Geometry: final body of the model. Coordinates: model frame, mm. A direction names the side the tool comes from. Give positions to 0.01 mm unless a question says otherwise; leave off trailing zeros. Write each loop counter-clockwise with the first axis right and the second up, starting at its lowest first coordinate (ties: lowest second). Pieces come first, ordered by that corner, then holes. Notation, with made-up numbers: M -35,-37 L -27,-37 A14 cw -27,-29 Z; hole C 31.25,26 d8. An arc over 180 degrees is marked long. Use a Markdown table: item, result. Add a question column.
(1) Material intervals for L1, parallel to Y at x = 0, z = 1.35; L2, parallel to Z at x = -14.5, y = 4.5; L3, parallel to X at y = 4, z = 0.3, sorted ascending.
(2) Cut plane B-B (y = -3.75). Output: boundary loops of the cut face in (x, z).
(3) Draft query along Y for faces 4 (the cylindrical face through (13.46, -1.36, 1.32)), 5 (the flat face through (0, -9, 1)), 6 (the flat face through (-11, 9, 1)). Return one class per face: released by +Y, released by -Y, zero draft, split by the parting line, or undercut.
(4) Pin query (flat end, axial travel): pin 1 Ø2.5 at (y, z) = (12.5, 2.5) entering from -X; pin 2 Ø1 at (y, z) = (7.5, 1.5) entering from +X; pin 3 Ø16 at (x, y) = (-6, -1) entering from +Z. Return the tip coordinate at first contact, or that it passes through.
(5) Reachability of faces 1 (the flat face through (8, 12, 2)), 2 (the flat face through (-12, 1.875, 1)), 3 (the flat face through (12, 9, 1)) from +Z, -Z, +X, -X, +Y, -Y: full face, straight path, thin tool, end or side. Return the list, or none.
(6) Cut plane D-D (y = 2.25). Output: boundary loops of the cut face in (x, z).
(7) Cut plane C-C (z = 1.6). State how many separate pieces and enclosed holes the cut face has, plus the area to 3 significant figures.
(8) Cut plane A-A (x = 0). Output: boundary loops of the cut face in (y, z).
```python
from build123d import *

# Parameters (mm, degrees)
F0_W     = 5
F0_H     = 3.75
F0_R     = 4.5
F1_DEPTH = 2.6
F2_W     = 16
F2_H     = 8.7
F3_DEPTH = 2
F4_R     = 4
F5_R     = 1.8
F6_R     = 2


with BuildPart() as f1:
    # F0 (on Top) → F1 (new body)
    with BuildSketch(Plane.XY):
        Polygon((17, -9), (17, 9), (8, 9), (8, 17.7), (-8, 17.7), (-8, 9), (-17, 9), (-17, -9), align=None)
        with Locations((-11.5, 0)):
            Rectangle(F0_W, F0_H, mode=Mode.SUBTRACT)
        Circle(F0_R, mode=Mode.SUBTRACT)
        with Locations((11.5, 0)):
            Rectangle(F0_W, F0_H, mode=Mode.SUBTRACT)
    extrude(amount=F1_DEPTH)

    # F2 (on face) → F3 (join)
    with BuildSketch(Plane.XY.offset(2.6)):
        with Locations((0, 13.35)):
            Rectangle(F2_W, F2_H)
    extrude(amount=F3_DEPTH)

    # F4
    f4_edges = [f1.edges().sort_by_distance(p)[0] for p in [
        (17, 9, 1.3),
        (17, -9, 1.3),
        (-17, 9, 1.3),
        (-17, -9, 1.3),
        (8, 17.7, 2.3),
        (-8, 17.7, 2.3),
    ]]
    fillet(f4_edges, radius=F4_R)

    # F5
    f5_edges = [f1.edges().sort_by_distance(p)[0] for p in [
        (0, 9, 4.6),
        (-14, 1.875, 1.3),
        (-14, -1.875, 1.3),
        (-9, 1.875, 1.3),
        (-9, -1.875, 1.3),
        (14, 1.875, 1.3),
        (9, 1.875, 1.3),
        (9, -1.875, 1.3),
        (14, -1.875, 1.3),
    ]]
    fillet(f5_edges, radius=F5_R)

    # F6
    f6_edges = [f1.edges().sort_by_distance(p)[0] for p in [
        (8, 9, 1.3),
        (-8, 9, 1.3),
    ]]
    fillet(f6_edges, radius=F6_R)


solid = f1.part
```
Answer list:
| question | item | result |
|---|---|---|
| 1 | L1 | -9 to -4.5, 4.5 to 17.7 |
| 1 | L2 | 0 to 2.6 |
| 1 | L3 | -17 to -2.06, 2.06 to 17 |
| 2 | outline | M -17,0 L -2.49,0 L -2.49,2.6 L -17,2.6 Z; M 2.49,0 L 17,0 L 17,2.6 L 2.49,2.6 Z |
| 3 | face 4 | undercut |
| 3 | face 5 | released by -Y |
| 3 | face 6 | released by +Y |
| 4 | pin 1 | x = -8 |
| 4 | pin 2 | x = 16.46 |
| 4 | pin 3 | z = 2.6 |
| 5 | face 1 | +Z, +X, +Y |
| 5 | face 2 | +Z, -Z |
| 5 | face 3 | +Z, -Z, +X, +Y |
| 6 | outline | M -17,0 L -3.9,0 L -3.9,2.6 L -17,2.6 Z; M 3.9,0 L 17,0 L 17,2.6 L 3.9,2.6 Z |
| 7 | separate pieces | 1 |
| 7 | enclosed holes | 3 |
| 7 | area | 637 mm² |
| 8 | outline | M -9,0 L -4.5,0 L -4.5,2.6 L -9,2.6 Z; M 4.5,0 L 17.7,0 L 17.7,4.6 L 10.8,4.6 A1.8 ccw 9,2.8 L 9,2.6 L 4.5,2.6 Z |
